```python
from build123d import *

# Parameters (mm, degrees)
F_3_5_3_5_DIAMETER_HOLE1_D = 3.5
CHAMFER1_SIZE              = 0.25


with BuildPart() as part:
    # Sketch2 → Revolve1 (revolve)
    with BuildSketch(Plane.XY):
        Polygon((-11, 0), (-1.75, 0), (-1.75, -3.2), (-2.85, -3.2), (-2.85, -6.2), (-4.4, -6.2), (-4.4, -2), (-11, -2), align=None)
    revolve(axis=Axis((0, 0, 0), (0, 1, 0)))

    # Ø3.5 (3.5) Diameter Hole1 (through all)
    with Locations(Plane(origin=(0, 0, 0), x_dir=(1, 0, 0), z_dir=(0, 1, 0))):
        with Locations((0, 8), (0, -8), (-8, 0), (8, 0)):
            Hole(F_3_5_3_5_DIAMETER_HOLE1_D / 2)

    # Chamfer1
    chamfer1_edges = [part.edges().sort_by_distance(p)[0] for p in [
        (11, 0, 0),
        (4.4, -6.2, 0),
        (11, -2, 0),
    ]]
    chamfer(chamfer1_edges, length=CHAMFER1_SIZE)


solid = part.part
```
For this review, take the finished solid that the model builds, in its own axes (mm). A direction names the side the tool comes from. Coordinates: 2 decimals unless noted, no trailing zeros. Loops run counter-clockwise (first coordinate to the right, second up) from the corner with the lowest first, then second, coordinate; pieces in that order, holes last. Notation, with made-up numbers: (15.5, 79.5) -> (70.5, 79.5) arc R20 ccw to (70.5, 94.5) -> close; hole circle Ø2 at (49, 67). An arc over 180 degrees is marked (long way). Return JSON: item names as keys, results as strings. Group by question number.
(1) Mouldability with a two-part tool opening along Z and no side actions: class faces 1 (the cylindrical face through (-1.617, -1.622, -0.67)), 2 (the flat face through (0, -2, -5)), 3 (the cylindrical face through (-4.197, -3.947, 1.322)) as pulls with the +Z half, pulls with the -Z half, needs draft (parallel to the pull), parting line crosses it, or undercut.
(2) Consider section B-B, the plane y = -1. Give the boundary of the cut face in (x, z).
(3) For pin 1 Ø3 at (x, z) = (8, 0) entering from +Y; pin 2 Ø6.5 at (x, z) = (0, 0) entering from -Y; pin 3 Ø1.5 at (x, y) = (-6.5, -1) entering from -Z; pin 4 Ø3 at (x, y) = (-4.5, -5.5) entering from -Z, all flat-tipped, find the tip position at first contact; note any pin that passes through.
(4) To check wall thickness, follow L1, parallel to Z at x = 0, y = -1.25; L2, parallel to Z at x = 0, y = -4.25; L3, parallel to Y at x = 0.25, z = -2.5. State the ranges of each line that lie inside material, in increasing order.
(5) Consider section A-A, the plane z = 0. Count the separate pieces of the cut face and the enclosed holes in it, plus the area to 3 significant figures.
(6) Tool access review of faces 4 (the cylindrical face through (0.228, -1.014, -9.735)), 5 (the flat face through (0, -3.2, -2)): name each direction out of +Z, -Z, +X, -X, +Y, -Y from which nothing blocks a thin tool from reaching the whole face with its end or side.
Results below:
{
 "1": {"face 1": "undercut", "face 2": "needs draft", "face 3": "parting line crosses it"},
 "2": {"outline": "circle Ø22 at (0, 0); hole circle Ø3.5 at (-8, 0); hole circle Ø3.5 at (0, -8); hole circle Ø3.5 at (0, 0); hole circle Ø3.5 at (0, 8); hole circle Ø3.5 at (8, 0)"},
 "3": {"pin 1": "passes through", "pin 2": "stops at y = -6.2", "pin 3": "stops at z = -9.38", "pin 4": "stops at z = -3.22"},
 "4": {"L1": "z = -11 to -9.75, -6.25 to -1.75, 1.75 to 6.25, 9.75 to 11", "L2": "z = -4.4 to -2.85, 2.85 to 4.4", "L3": "y = -3.2 to 0"},
 "5": {"separate pieces": "4", "enclosed holes": "0", "area": "38.5 mm2"},
 "6": {"face 4": "+Y, -Y", "face 5": "-Y"}
}
